from build123d import *

# Parameters (mm, degrees)
BOSS_EXTRUDE1_DEPTH = 56
SKETCH14_W          = 42.4
SKETCH14_H          = 42.4
CUT_EXTRUDE1_DEPTH  = 56
CHAMFER1_SIZE       = 3.5
FILLET1_R           = 10
SKETCH16_W          = 12.4
SKETCH16_H          = 23
CUT_EXTRUDE3_DEPTH  = 95.009532523
CUT_EXTRUDE4_REACH  = 93.39
SKETCH17_W          = 15.453545708
SKETCH17_H          = 18
FILLET4_R           = 15


with BuildPart() as part:
    # Sketch1 → Boss-Extrude1 (new body)
    with BuildSketch(Plane.XY):
        with BuildLine():
            Line((13.02, -7.9417418), (17.7, -7.9417418))
            Line((17.7, -7.9417418), (17.7, 70.02))
            Line((17.7, 70.02), (-10.566443095, 70.02))
            Line((-10.566443095, 70.02), (-10.566443095, 13.02))
            Line((-10.566443095, 13.02), (-5.317126718, 13.02))
            Line((-5.317126718, 13.02), (-4.287512407, 13.02))
            ThreePointArc((-4.287512407, 13.02), (-3.319474451, 12.619025549), (-2.9185, 11.650987593))
            Line((-2.9185, 11.650987593), (-2.9185, 11.539212407))
            ThreePointArc((-2.9185, 11.539212407), (-3.319474451, 10.571174451), (-4.287512407, 10.1702))
            Line((-4.287512407, 10.1702), (-6.476788598, 10.1702))
            ThreePointArc((-6.476788598, 10.1702), (-7.136510935, 9.729114651), (-6.981020848, 8.950903446))
            Line((-6.981020848, 8.950903446), (-3.672257405, 5.649701928))
            ThreePointArc((-3.672257405, 5.649701928), (-2.746830644, 5.032499411), (-1.655778399, 4.8158))
            Line((-1.655778399, 4.8158), (1.655778399, 4.8158))
            ThreePointArc((1.655778399, 4.8158), (2.746830644, 5.032499411), (3.672257405, 5.649701928))
            Line((3.672257405, 5.649701928), (6.981020848, 8.950903446))
            ThreePointArc((6.981020848, 8.950903446), (7.136510935, 9.729114651), (6.476788598, 10.1702))
            Line((6.476788598, 10.1702), (4.287512407, 10.1702))
            ThreePointArc((4.287512407, 10.1702), (3.319474451, 10.571174451), (2.9185, 11.539212407))
            Line((2.9185, 11.539212407), (2.9185, 11.650987593))
            ThreePointArc((2.9185, 11.650987593), (3.319474451, 12.619025549), (4.287512407, 13.02))
            Line((4.287512407, 13.02), (6.332886163, 13.02))
            Line((6.332886163, 13.02), (10.562594215, 13.019824354))
            ThreePointArc((10.562594215, 13.019824354), (12.303594776, 12.313982883), (13.019956614, 10.577284622))
            Line((13.019956614, 10.577284622), (13.02, 4.287469289))
            ThreePointArc((13.02, 4.287469289), (12.619025549, 3.319431332), (11.650987593, 2.918456882))
            Line((11.650987593, 2.918456882), (11.539212407, 2.918456882))
            ThreePointArc((11.539212407, 2.918456882), (10.571174451, 3.319431332), (10.1702, 4.287469289))
            Line((10.1702, 4.287469289), (10.1702, 6.402089023))
            ThreePointArc((10.1702, 6.402089023), (9.733877283, 7.055496588), (8.963146507, 6.90287605))
            Line((8.963146507, 6.90287605), (5.667020993, 3.614283579))
            ThreePointArc((5.667020993, 3.614283579), (5.046449321, 2.687255303), (4.8285, 1.593185507))
            Line((4.8285, 1.593185507), (4.8285, -1.593185507))
            ThreePointArc((4.8285, -1.593185507), (5.046449321, -2.687255303), (5.667020993, -3.614283579))
            Line((5.667020993, -3.614283579), (8.963146507, -6.90287605))
            ThreePointArc((8.963146507, -6.90287605), (9.733877283, -7.055496588), (10.1702, -6.402089023))
            Line((10.1702, -6.402089023), (10.1702, -4.287469289))
            ThreePointArc((10.1702, -4.287469289), (10.571174451, -3.319431332), (11.539212407, -2.918456882))
            Line((11.539212407, -2.918456882), (11.650987593, -2.918456882))
            ThreePointArc((11.650987593, -2.918456882), (12.619025549, -3.319431332), (13.02, -4.287469289))
            Line((13.02, -4.287469289), (13.02, -5.3170836))
            Line((13.02, -5.3170836), (13.02, -7.9417418))
        make_face()
    extrude(amount=BOSS_EXTRUDE1_DEPTH)

    # Sketch14 → Cut-Extrude1 (cut)
    with BuildSketch(Plane(origin=(17.7, 0, 0), x_dir=(0, 0, -1), z_dir=(1, 0, 0))):
        with Locations((-28, 42.22)):
            Rectangle(SKETCH14_W, SKETCH14_H)
    extrude(amount=-CUT_EXTRUDE1_DEPTH, mode=Mode.SUBTRACT)

    # Chamfer1
    chamfer1_edges = [part.edges().sort_by_distance(p)[0] for p in [
        (3.566778452, 21.02, 49.2),
        (3.566778452, 63.42, 49.2),
        (3.566778452, 63.42, 6.8),
        (3.566778452, 21.02, 6.8),
    ]]
    chamfer(chamfer1_edges, length=CHAMFER1_SIZE)

    # Fillet1
    fillet1_edges = [part.edges().sort_by_distance(p)[0] for p in [
        (3.566778452, 70.02, 56),
        (3.566778452, 70.02, 0),
    ]]
    fillet(fillet1_edges, radius=FILLET1_R)

    # Sketch16 → Cut-Extrude3 (cut, through all)
    with BuildSketch(Plane(origin=(17.7, 0, 0), x_dir=(0, 0, -1), z_dir=(1, 0, 0))):
        with Locations((-49.8, 3.5582582)):
            Rectangle(SKETCH16_W, SKETCH16_H)
    extrude(amount=-CUT_EXTRUDE3_DEPTH, mode=Mode.SUBTRACT)

    # Sketch17 → Cut-Extrude4 (cut, up to next)
    with BuildSketch(Plane.XY.offset(56), mode=Mode.PRIVATE) as cut_extrude4_sk1:
        with Locations((-5.893215949, 42.22)):
            Rectangle(SKETCH17_W, SKETCH17_H)
    cut_extrude4_tool1 = extrude(cut_extrude4_sk1.sketch, amount=-CUT_EXTRUDE4_REACH, mode=Mode.PRIVATE) & part.part
    add(cut_extrude4_tool1.solids().sort_by_distance((-5.893216, 42.22, 56))[0], mode=Mode.SUBTRACT)

    # Fillet4
    # the kernel refuses this fillet: 15 mm, written as the material it takes off along each edge
    with BuildSketch(Plane(origin=(54.632370625, 15.0582582, 56), x_dir=(0, 1, 0), z_dir=(-1, 0, 0))) as fillet4_piece_1:
        with BuildLine():
            CenterArc((14.77294825, 15), FILLET4_R, 189.98168298, 80.01831702)
            Line((0, 12.4), (-0.295458965, 12.348))
            ThreePointArc((-0.295458965, 12.348), (-0.3, 6.2), (-0.3, 0))
            Line((-0.3, 0), (0, -0.3))
            Line((0, -0.3), (14.77294825, -0.3))
            Line((14.77294825, -0.3), (14.77294825, 0))
        make_face()
    extrude(amount=102.131184346, mode=Mode.SUBTRACT)


solid = part.part
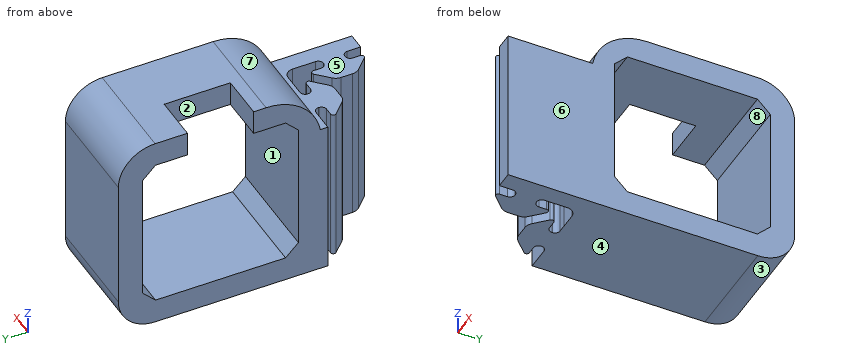
Read the model definition and answer for the solid it produces. Units are mm, in the model's axes. Face numbers are marked on the shaded views. A direction names the side the tool comes from. Round coordinates to 2 decimals unless told otherwise and drop trailing zeros. Write each loop counter-clockwise with the first axis right and the second up, starting at its lowest first coordinate (ties: lowest second). Pieces come first, ordered by that corner, then holes. Notation, with made-up numbers: (78, 65) - (104, 65) arc R26 ccw to (104, 93) - close; hole circle Ø10 at (79, 55). An arc over 180 degrees is marked (long way). Use a Markdown table: item, result.
(1) Each of these flat-tipped pins is pushed along its axis until it touches: pin 1 Ø2 at (x, z) = (-4.5, 51.5) entering from -Y; pin 2 Ø3.5 at (x, z) = (0.5, 12.5) entering from -Y; pin 3 Ø7 at (y, z) = (7, 26.5) entering from -X. Where does it stop, or does it pass through?
Reported:
| item | result |
|---|---|
| pin 1 | y = 18.22 |
| pin 2 | y = 4.82 |
| pin 3 | x = -7.19 |
(2) The mould has two halves that part along Z. Classify the marked faces 6, 7 and 8: released by +Z, released by -Z, zero draft, split by the parting line, or undercut.
Reported:
| item | result |
|---|---|
| face 6 | zero draft |
| face 7 | released by +Z |
| face 8 | undercut |
(3) The part is cut by section C-C (x = 14.5). Write down the section's boundary in (y, z), then the cut area to 3 significant figures.
Reported:
| item | result |
|---|---|
| outline | (-7.94, 0) - (60.02, 0) arc R10 ccw to (70.02, 10) - (70.02, 46) arc R10 ccw to (60.02, 56) - (29.83, 56) arc R15 ccw to (15.06, 43.6) - (-7.94, 43.6) - close; hole (21.02, 10.3) - (24.52, 6.8) - (59.92, 6.8) - (63.42, 10.3) - (63.42, 45.7) - (59.92, 49.2) - (24.52, 49.2) - (21.02, 45.7) - close |
| area | 2,220 mm2 |
(4) The part is cut by section A-A (y = 41). Write down the section's boundary in (x, z), then the cut area to 3 significant figures.
Reported:
| item | result |
|---|---|
| outline | (-10.57, 0) - (17.7, 0) - (17.7, 6.8) - (-10.57, 6.8) - close; (1.83, 49.2) - (17.7, 49.2) - (17.7, 56) - (1.83, 56) - close |
| area | 300 mm2 |
(5) The part is cut by section D-D (y = 65). Write down the section's boundary in (x, z).
Reported:
| item | result |
|---|---|
| outline | (-10.57, 1.33) - (17.7, 1.33) - (17.7, 54.67) - (-10.57, 54.67) - close |
(6) The part is cut by section B-B (x = 0). Write down the section's boundary in (y, z).
Reported:
| item | result |
|---|---|
| outline | (4.82, 0) - (60.02, 0) arc R10 ccw to (70.02, 10) - (70.02, 46) arc R10 ccw to (60.02, 56) - (51.22, 56) - (51.22, 49.2) - (59.92, 49.2) - (63.42, 45.7) - (63.42, 10.3) - (59.92, 6.8) - (24.52, 6.8) - (21.02, 10.3) - (21.02, 45.7) - (24.52, 49.2) - (33.22, 49.2) - (33.22, 56) - (29.83, 56) arc R15 ccw to (15.06, 43.6) - (4.82, 43.6) - close |
(7) Which of the six approach directions +Z, -Z, +X, -X, +Y, -Y give full straight-line access (tool end or side, diameter ignored) to the marked faces 1, 2, 3, 4 and 5?
Reported:
| item | result |
|---|---|
| face 1 | +X, -X |
| face 2 | +Z, -X |
| face 3 | -Z, +X, -X, +Y |
| face 4 | -Z, +X, -X, +Y, -Y |
| face 5 | +Z, +X, -X, -Y |
(8) Straight lines are drawn through the part: line 1 along Z through (x, y) = (3.75, 56); line 2 along Y through (x, z) = (16, 39.5); line 3 along Y through (x, z) = (1.5, 39.5). For each, find the intervals that lie inside material, in ascending order. Write a range as [from, to].
Reported:
| item | result |
|---|---|
| line 1 | [0, 6.8], [49.2, 56] |
| line 2 | [-7.94, 21.02], [63.42, 70.02] |
| line 3 | [4.82, 21.02], [63.42, 70.02] |
